Read the model definition and answer for the solid it produces. Units are mm, in the model's axes. Coordinates: 2 decimals unless noted, no trailing zeros. Loops run counter-clockwise (first coordinate to the right, second up) from the corner with the lowest first, then second, coordinate; pieces in that order, holes last. Notation, with made-up numbers: (88, -12) -> (114, -12) arc R22 cw to (114, 3) -> close; hole circle Ø4 at (-2, 68). An arc over 180 degrees is marked (long way). Answer in a Markdown table with one row per item.
Autodesk Inventor part; units mm, degrees
ref_plane "YZ Plane" through (0, 0, 0) normal (1, 0, 0) x (0, 1, 0)
ref_plane "XZ Plane" through (0, 0, 0) normal (0, 1, 0) x (-1, 0, 0)
ref_plane "XY Plane" through (0, 0, 0) normal (0, 0, 1) x (1, 0, 0)
sketch "Sketch1" plane through (0, 0, 0) normal (0, 0, 1) x (1, 0, 0)
  line L0 (0, 0) -> (62.2, 0)
  line L1 (62.2, 0) -> (62.2, 54.6)
  line L2 (62.2, 54.6) -> (0, 54.6)
  line L3 (0, 54.6) -> (0, 0)
  line L4 (1, 54.6) -> (1, 0) construction
  line L5 (0, 1) -> (62.2, 1) construction
  line L6 (61.2, 0) -> (61.2, 54.6) construction
  line L7 (0, 53.6) -> (62.2, 53.6) construction
  circle A0 centre (2.5, 52.1) radius 1.5
  circle A1 centre (59.7, 52.1) radius 1.5
  circle A2 centre (2.5, 2.5) radius 1.5
  circle A3 centre (59.7, 2.5) radius 1.5
  point P0 (33.2, 0)
  dimension "d0" = 62.2
  dimension "d1" = 54.6
  dimension "d2" = 29
  dimension "d3" = 1
  dimension "d4" = 1
  dimension "d5" = 1
  dimension "d6" = 1
  dimension "d7" = 3
extrude "Extrusion1" add sketch "Sketch1" along normal blind 16.9
ref_plane "Work Plane1" through (0, 0, 16.9) normal (0, 0, 1) x (1, 0, 0)
sketch "Sketch2" plane through (0, 0, 16.9) normal (0, 0, 1) x (1, 0, 0)
  line L0 (0, 0) -> (62.2, 0)
  line L1 (29.4, 0) -> (37, 0)
  line L2 (37, 0) -> (37, 9.2)
  line L3 (37, 9.2) -> (29.4, 9.2)
  line L4 (29.4, 9.2) -> (29.4, 0)
  point P0 (33.2, 0)
  dimension "d11" = 29
  dimension "d12" = 7.6
  dimension "d13" = 9.2
extrude "Extrusion2" add sketch "Sketch2" along normal blind 2.5
equation "\"d4\" = d3"
equation "\"d5\" = d3"
equation "\"d6\" = d3"
properties part number "board_rev0"
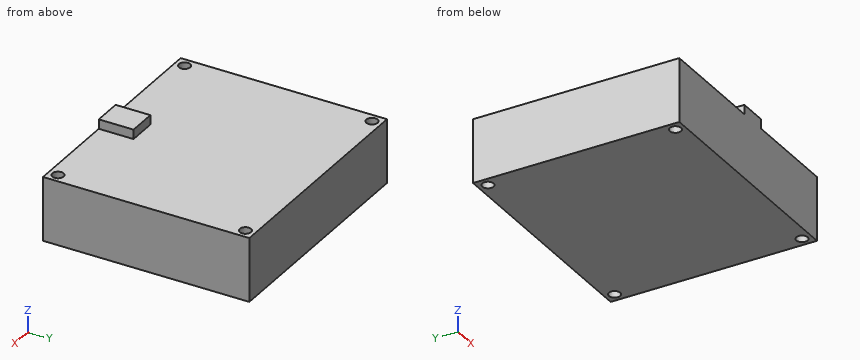
1. Given pin 1 Ø1.2 at (y, z) = (6.5, 18) entering from -X; pin 2 Ø5 at (x, y) = (26, 37) entering from +Z, each flat-ended and moving along its own axis, determine where each tip first touches the part or whether it passes through.
A:
| item | result |
|---|---|
| pin 1 | stops at x = 29.4 |
| pin 2 | stops at z = 16.9 |
2. Find the intervals of material crossed by probe 1 along Y at (x, z) = (2.5, 4.5); probe 2 along Z at (x, y) = (10, 29.5); probe 3 along Y at (x, z) = (33, 18.5), in increasing order.
A:
| item | result |
|---|---|
| probe 1 | y = 0 to 1, 4 to 50.6, 53.6 to 54.6 |
| probe 2 | z = 0 to 16.9 |
| probe 3 | y = 0 to 9.2 |
3. A cutting plane is placed at A-A on y = 2.5. Give the vertices of the cut face in (x, z).
A:
| item | result |
|---|---|
| outline | (0, 0) -> (1, 0) -> (1, 16.9) -> (0, 16.9) -> close; (4, 0) -> (58.2, 0) -> (58.2, 16.9) -> (37, 16.9) -> (37, 19.4) -> (29.4, 19.4) -> (29.4, 16.9) -> (4, 16.9) -> close; (61.2, 0) -> (62.2, 0) -> (62.2, 16.9) -> (61.2, 16.9) -> close |
4. A cutting plane is placed at B-B on x = 2.5. Give the vertices of the cut face in (y, z), and give its area (3 significant figures).
A:
| item | result |
|---|---|
| outline | (0, 0) -> (1, 0) -> (1, 16.9) -> (0, 16.9) -> close; (4, 0) -> (50.6, 0) -> (50.6, 16.9) -> (4, 16.9) -> close; (53.6, 0) -> (54.6, 0) -> (54.6, 16.9) -> (53.6, 16.9) -> close |
| area | 821 mm2 |
5. A cutting plane is placed at C-C on y = 52.1. Give the vertices of the cut face in (x, z).
A:
| item | result |
|---|---|
| outline | (0, 0) -> (1, 0) -> (1, 16.9) -> (0, 16.9) -> close; (4, 0) -> (58.2, 0) -> (58.2, 16.9) -> (4, 16.9) -> close; (61.2, 0) -> (62.2, 0) -> (62.2, 16.9) -> (61.2, 16.9) -> close |
6. A cutting plane is placed at D-D on x = 41. Give the vertices of the cut face in (y, z).
A:
| item | result |
|---|---|
| outline | (0, 0) -> (54.6, 0) -> (54.6, 16.9) -> (0, 16.9) -> close |
